For this review, use the dimensioned drawing (mm, ordinates from the lowest corner) and the shaded views. A direction names the side the tool comes from. Round coordinates to 2 decimals unless told otherwise and drop trailing zeros. Order: outer loops, then holes, each group sorted by start corner. A loop starts at its lowest first (then second) coordinate and runs counter-clockwise, first axis right, second up. Notation, with made-up numbers: (60, 3) -> (83, 3) arc R29 ccw to (83, 31) -> close; hole circle Ø5 at (-31, 73.5). An arc over 180 degrees is marked (long way). Answer in a Markdown table with one row per item.
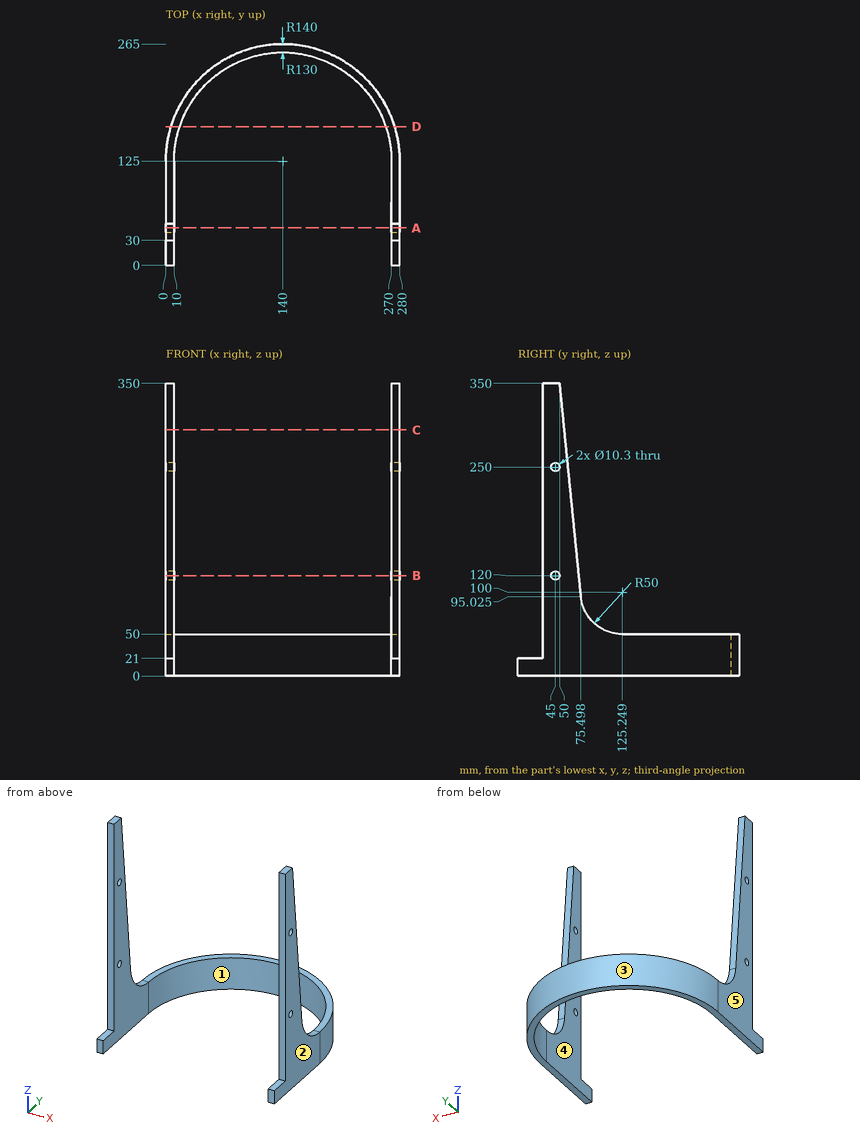
Q1. Take a section at B-B, the plane z = 120. Write out the cut boundary in (x, y), then the cut area to 3 significant figures.
Answer key:
| item | result |
|---|---|
| outline | (0, 30) -> (10, 30) -> (10, 39.85) -> (0, 39.85) -> close; (0, 50.15) -> (10, 50.15) -> (10, 73) -> (0, 73) -> close; (270, 30) -> (280, 30) -> (280, 39.85) -> (270, 39.85) -> close; (270, 50.15) -> (280, 50.15) -> (280, 73) -> (270, 73) -> close |
| area | 654 mm^2 |
Q2. Take a section at A-A, the plane y = 45. Write out the cut boundary in (x, z).
Answer key:
| item | result |
|---|---|
| outline | (0, 0) -> (10, 0) -> (10, 114.85) -> (0, 114.85) -> close; (0, 125.15) -> (10, 125.15) -> (10, 244.85) -> (0, 244.85) -> close; (0, 255.15) -> (10, 255.15) -> (10, 350) -> (0, 350) -> close; (270, 0) -> (280, 0) -> (280, 114.85) -> (270, 114.85) -> close; (270, 125.15) -> (280, 125.15) -> (280, 244.85) -> (270, 244.85) -> close; (270, 255.15) -> (280, 255.15) -> (280, 350) -> (270, 350) -> close |
Q3. Tool access review of the marked faces 4 and 5: name each direction out of +Z, -Z, +X, -X, +Y, -Y from which nothing blocks a thin tool from reaching the whole face with its end or side.
Answer key:
| item | result |
|---|---|
| face 4 | +Z, -Z, -Y |
| face 5 | +Z, -Z, -X, +Y, -Y |
Q4. Take a section at C-C, the plane z = 294.5. Write out the cut boundary in (x, y).
Answer key:
| item | result |
|---|---|
| outline | (0, 30) -> (10, 30) -> (10, 55.55) -> (0, 55.55) -> close; (270, 30) -> (280, 30) -> (280, 55.55) -> (270, 55.55) -> close |
Q5. To check wall thickness, follow probe 1 along Z at (x, y) = (5, 45); probe 2 along X at (y, z) = (74.5, 102.5); probe 3 along Y at (x, z) = (207, 16.5) (1 decimal). State the ranges of each line that lie inside material, in increasing order.
Answer key:
| item | result |
|---|---|
| probe 1 | z = 0 to 114.85, 125.15 to 244.85, 255.15 to 350 |
| probe 2 | x = 0 to 10, 270 to 280 |
| probe 3 | y = 236.4 to 247.9 |
Q6. Take a section at D-D, the plane y = 166. Write out the cut boundary in (x, z) (1 decimal), then the cut area to 3 significant figures.
Answer key:
| item | result |
|---|---|
| outline | (6.1, 0) -> (16.6, 0) -> (16.6, 50) -> (6.1, 50) -> close; (263.4, 0) -> (273.9, 0) -> (273.9, 50) -> (263.4, 50) -> close |
| area | 1,050 mm^2 |
Q7. The part is to be moulded in two halves that separate along X. For the marked faces 1, 2 and 3, say which applies: +X half, -X half, draft (parallel to the pull), parting line (faces both ways), or undercut.
Answer key:
| item | result |
|---|---|
| face 1 | undercut |
| face 2 | +X half |
| face 3 | parting line |
Q8. Clearance check with flat-ended pins moving along their axes: pin 1 Ø6 at (x, z) = (210, 45) entering from +Y; pin 2 Ø3 at (x, y) = (276.5, 8) entering from +Z; pin 3 Ø5 at (x, z) = (229.5, 51) entering from -Y (1 decimal); pin 4 Ø6 at (y, z) = (45, 250) entering from -X. State where each tip first meets the part, or that it passes through.
Answer key:
| item | result |
|---|---|
| pin 1 | stops at y = 247.93 |
| pin 2 | stops at z = 21 |
| pin 3 | stops at y = 217.1 |
| pin 4 | passes through |
